For this review, take the finished solid that the model builds, in its own axes (mm). Round coordinates to 2 decimals unless told otherwise and drop trailing zeros. Order: outer loops, then holes, each group sorted by start corner. A loop starts at its lowest first (then second) coordinate and runs counter-clockwise, first axis right, second up.
```python
from build123d import *

# Parameters (mm, degrees)
F1_DEPTH = 25.4
F2_DEPTH = 25.4
F3_DEPTH = 76.2


with BuildPart() as f1:
    # F0 (on Front) → F1 (new body)
    with BuildSketch(Plane.XZ):
        Polygon((-10.2298520505, 29.5050740242), (-65.3136447072, 0), (-10.2298520505, 0), align=None)
        Polygon((-10.2298520505, 29.5050740242), (-10.2298520505, 0), (44.8539443314, 0), align=None)
    extrude(amount=F1_DEPTH)

    # F2 (add): a face of the model
    f2_faces = [f1.faces().sort_by_distance(p)[0] for p in [
        (-10.2298508088, -25.4, 9.8350246747),
    ]]
    extrude(f2_faces, amount=F2_DEPTH)

    # F3 (add): a face of the model
    f3_faces = [f1.faces().sort_by_distance(p)[0] for p in [
        (-10.2298508088, -50.8, 9.8350246747),
    ]]
    extrude(f3_faces, amount=F3_DEPTH)


solid = f1.part
```
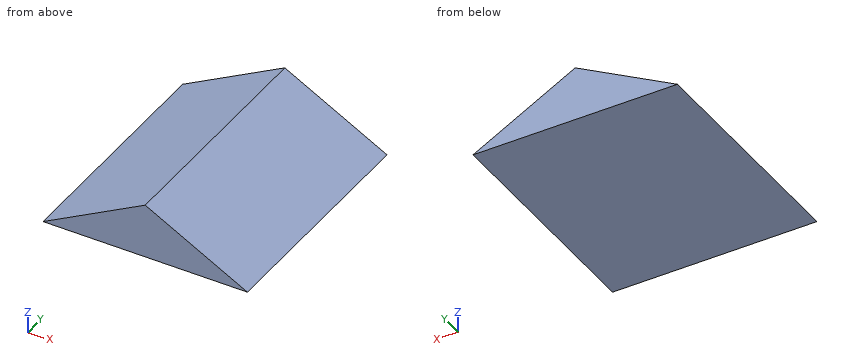
Q1. Wall thickness on line 1 (Z direction, x = -13.5, y = -115); line 2 (X direction, y = -16.5, z = 11.25); line 3 (Z direction, x = 18, y = -40.5): over which ranges is each line inside the solid? List them lowest first.
Q2. Take a section at A-A, the plane y = -106. State the section outline as (x, z) points, plus the area to 3 significant figures.
Q3. Take a section at B-B, the plane z = 12. State the section outline as (x, y) points, plus the area to 3 significant figures.
Q4. Take a section at C-C, the plane x = 11. State the section outline as (y, z) points, plus the area to 3 significant figures.
Q5. Clearance check with flat-ended pins moving along their axes: pin 1 (2 mm diameter, centred on y = -51, z = 26, fed in from +X); pin 2 (4 mm diameter, centred on y = -37.5, z = 19.5, fed in from +X); pin 3 (1.5 mm diameter, centred on y = -16, z = 10.5, fed in from -X). State where each tip first meets the part, or that it passes through.
Working result:
1. line 1: z = 0 to 27.75
1. line 2: x = -44.31 to 23.85
1. line 3: z = 0 to 14.38
2. outline: (-65.31, 0) - (44.85, 0) - (-10.23, 29.51) - close
2. area: 1,630 mm2
3. outline: (-42.91, -127) - (22.45, -127) - (22.45, 0) - (-42.91, 0) - close
3. area: 8,300 mm2
4. outline: (-127, 0) - (0, 0) - (0, 18.13) - (-127, 18.13) - close
4. area: 2,300 mm2
5. pin 1: stops at x = -1.82
5. pin 2: stops at x = 12.18
5. pin 3: stops at x = -47.11
